Here's how the part is built. I have some questions about the finished solid (model axes, mm). A direction names the side the tool comes from. Coordinates: 2 decimals unless noted, no trailing zeros. Order: outer loops, then holes, each group sorted by start corner. A loop starts at its lowest first (then second) coordinate and runs counter-clockwise, first axis right, second up. Notation, with made-up numbers: (47.25, 9.25) - (56.25, 9.25) arc R34 cw to (56.25, 46.25) - close; hole circle Ø3 at (29, 36). An arc over 180 degrees is marked (long way). Answer in a Markdown table with one row per item. Add a question column.
Item 1: I want a section at B-B (x = 0). Please give me the cut outline in (y, z) (1 decimal), plus the area to 3 significant figures.
Item 2: Will these pins go through, and if not, where does the flat tip stop? pin 1 Ø2.5 at (x, z) = (0, -18.415) entering from +Y; pin 2 Ø4 at (x, z) = (20.64, 0) entering from +Y; pin 3 Ø3.5 at (x, z) = (15.95, 9.21) entering from -Y; pin 4 Ø5 at (y, z) = (7, 5) entering from +X.
Item 3: On a 3-axis mill with a long thin cutter (end or side, diameter ignored), from which of +Z, -Z, +X, -X, +Y, -Y can I reach the whole of each face in a straight line? I mean faces 4 (the cylindrical face through (-24.698, 6.63, -0.179)), 5 (the flat face through (0, 9.588, 12)). Say none if no direction works.
Item 4: If I drill on line 1 along X through (y, z) = (2.8, 0); line 2 along Z through (x, y) = (0, 8.5) (1 decimal); line 3 along Z through (x, y) = (-2.5, 5), over which ranges is the centre line in solid material (lowest first)? Write a range as from..to.
Item 5: I want a section at C-C (z = -6). Please give me the cut outline in (x, y).
Item 6: I want a section at A-A (z = 0). Please give me the cut outline in (x, y), plus the area to 3 significant figures.
Item 7: Thinking about a two-plate mould opening in X: for faces 1 (the cylindrical face through (-1.323, 4.727, -10.074)), 2 (the flat face through (0, 0, 12)), 3 (the cylindrical face through (-6.024, 4.727, 27.127)), which applies, +X half, -X half, draft (parallel to the pull), parting line (faces both ways), or undercut?
Item 8: I want a section at D-D (y = 5). Please give me the cut outline in (x, z) (1 decimal), plus the area to 3 significant figures.
```python
from build123d import *

# Parameters (mm, degrees)
SKETCH1_R               = 27.7876
SKETCH1_R_2             = 10.16
RING_DEPTH              = 9.5885
SKETCH2_R               = 1.5
ROBOT_SIDE1_HOLES_DEPTH = 10.5885
ROBOT_SIDE_CHAMFER_SIZE = 2.4
SKETCH3_R               = 1.838724863
TOOL_SIDE_HOLES_DEPTH   = 10.5885
SKETCH4_R               = 4.064
TOOL_SIDE_INSET_DEPTH   = 6


with BuildPart() as part:
    # Sketch1 → Ring (new body)
    with BuildSketch(Plane(origin=(0, 0, 0), x_dir=(1, 0, 0), z_dir=(0, 1, 0))):
        Circle(SKETCH1_R)
        Circle(SKETCH1_R_2, mode=Mode.SUBTRACT)
    extrude(amount=RING_DEPTH)

    # Sketch2 → Robot Side1 - Holes (cut, through all)
    with BuildSketch(Plane(origin=(0, 9.5885, 0), x_dir=(1, 0, 0), z_dir=(0, 1, 0))):
        with Locations((0, 18.415)):
            Circle(SKETCH2_R)
        with Locations((15.947857811, -9.2075)):
            Circle(SKETCH2_R)
        with Locations((-15.947857811, -9.2075)):
            Circle(SKETCH2_R)
    extrude(amount=-ROBOT_SIDE1_HOLES_DEPTH, mode=Mode.SUBTRACT)

    # Robot Side - Chamfer
    robot_side_chamfer_edges = [part.edges().sort_by_distance(p)[0] for p in [
        (-1.5, 0, -18.415),
        (14.447857811, 0, 9.2075),
        (-17.447857811, 0, 9.2075),
    ]]
    chamfer(robot_side_chamfer_edges, length=ROBOT_SIDE_CHAMFER_SIZE)

    # Sketch3 → Tool Side - Holes (cut, through all)
    with BuildSketch(Plane(origin=(0, 9.5885, 0), x_dir=(1, 0, 0), z_dir=(0, 1, 0))):
        with Locations((20.6375, 0)):
            Circle(SKETCH3_R)
        with Locations((0, -20.6375)):
            Circle(SKETCH3_R)
        with Locations((-20.6375, 0)):
            Circle(SKETCH3_R)
    extrude(amount=-TOOL_SIDE_HOLES_DEPTH, mode=Mode.SUBTRACT)

    # Sketch4 → Tool Side - Inset (cut)
    with BuildSketch(Plane(origin=(0, 9.5885, 0), x_dir=(1, 0, 0), z_dir=(0, 1, 0))):
        with Locations((-20.6375, 0)):
            Circle(SKETCH4_R)
        with Locations((0, -20.6375)):
            Circle(SKETCH4_R)
        with Locations((20.6375, 0)):
            Circle(SKETCH4_R)
    extrude(amount=-TOOL_SIDE_INSET_DEPTH, mode=Mode.SUBTRACT)


solid = part.part
```
Values follow:
| question | item | result |
|---|---|---|
| 1 | outline | (0, -27.8) - (9.6, -27.8) - (9.6, -19.9) - (2.4, -19.9) - (0, -22.3) - close; (0, -14.5) - (2.4, -16.9) - (9.6, -16.9) - (9.6, -10.2) - (0, -10.2) - close; (0, 10.2) - (9.6, 10.2) - (9.6, 16.6) - (3.6, 16.6) - (3.6, 18.8) - (0, 18.8) - close; (0, 22.5) - (3.6, 22.5) - (3.6, 24.7) - (9.6, 24.7) - (9.6, 27.8) - (0, 27.8) - close |
| 1 | area | 242 mm^2 |
| 2 | pin 1 | passes through |
| 2 | pin 2 | stops at y = 3.59 |
| 2 | pin 3 | stops at y = 2.15 |
| 2 | pin 4 | stops at x = 27.67 |
| 3 | face 4 | +Y |
| 3 | face 5 | +Z, -Z, +X, -X, +Y |
| 4 | line 1 | x = -27.79..-22.48, -18.8..-10.16, 10.16..18.8, 22.48..27.79 |
| 4 | line 2 | z = -27.8..-19.9, -16.9..-10.2, 10.2..16.6, 24.7..27.8 |
| 4 | line 3 | z = -27.67..-9.85, 9.85..17.43, 23.84..27.67 |
| 5 | outline | (-27.13, 0) - (-8.2, 0) - (-8.2, 9.59) - (-27.13, 9.59) - close; (8.2, 0) - (27.13, 0) - (27.13, 9.59) - (8.2, 9.59) - close |
| 6 | outline | (-27.79, 0) - (-22.48, 0) - (-22.48, 3.59) - (-24.7, 3.59) - (-24.7, 9.59) - (-27.79, 9.59) - close; (-18.8, 0) - (-10.16, 0) - (-10.16, 9.59) - (-16.57, 9.59) - (-16.57, 3.59) - (-18.8, 3.59) - close; (10.16, 0) - (18.8, 0) - (18.8, 3.59) - (16.57, 3.59) - (16.57, 9.59) - (10.16, 9.59) - close; (22.48, 0) - (27.79, 0) - (27.79, 9.59) - (24.7, 9.59) - (24.7, 3.59) - (22.48, 3.59) - close |
| 6 | area | 214 mm^2 |
| 7 | face 1 | undercut |
| 7 | face 2 | draft |
| 7 | face 3 | parting line |
| 8 | outline | circle Ø55.6 at (0, 0); hole circle Ø8.1 at (-20.6, 0); hole circle Ø3 at (-15.9, 9.2); hole circle Ø20.3 at (0, 0); hole circle Ø8.1 at (0, 20.6); hole circle Ø3 at (0, -18.4); hole circle Ø3 at (15.9, 9.2); hole circle Ø8.1 at (20.6, 0) |
| 8 | area | 1,920 mm^2 |
